Here's how the part is built. I have some questions about the finished solid (model axes, mm). Face numbers are marked on the shaded views. A direction names the side the tool comes from. Give positions to 0.01 mm unless a question says otherwise; leave off trailing zeros. Write each loop counter-clockwise with the first axis right and the second up, starting at its lowest first coordinate (ties: lowest second). Pieces come first, ordered by that corner, then holes. Notation, with made-up numbers: (16, 21) -> (32, 21) arc R26 ccw to (32, 49) -> close; hole circle Ø10 at (33.25, -8.5). An arc over 180 degrees is marked (long way). Return JSON: item names as keys, results as strings.
from build123d import *

# Parameters (mm, degrees)
SKETCH1_R               = 10
BOSS_EXTRUDE1_DEPTH     = 115
SKETCH2_R               = 5
BOSS_EXTRUDE2_DEPTH     = 25
SKETCH3_R               = 5
CUT_EXTRUDE1_DEPTH      = 110
SKETCH4_R               = 2.5
CUT_EXTRUDE2_DEPTH      = 11
CUT_EXTRUDE2_DEPTH_BACK = 11
SKETCH5_R               = 10
BOSS_EXTRUDE3_DEPTH     = 22
SKETCH6_W               = 21
SKETCH6_H               = 21
BOSS_EXTRUDE4_DEPTH     = 8
SKETCH7_W               = 21
SKETCH7_H               = 21
BOSS_EXTRUDE5_DEPTH     = 2
SKETCH8_R               = 5
SKETCH8_R_2             = 4
CUT_EXTRUDE3_DEPTH      = 2
SKETCH9_R               = 1.545135807
CUT_EXTRUDE4_DEPTH      = 2


with BuildPart() as part:
    # Sketch1 → Boss-Extrude1 (new body)
    with BuildSketch(Plane.XY):
        Circle(SKETCH1_R)
    extrude(amount=BOSS_EXTRUDE1_DEPTH)

    # Sketch2 → Boss-Extrude2 (add)
    with BuildSketch(Plane(origin=(0, 0, 0), x_dir=(-1, 0, 0), z_dir=(0, 0, -1))):
        Circle(SKETCH2_R)
    extrude(amount=BOSS_EXTRUDE2_DEPTH)

    # Sketch3 → Cut-Extrude1 (cut)
    with BuildSketch(Plane.XY.offset(115)):
        Circle(SKETCH3_R)
    extrude(amount=-CUT_EXTRUDE1_DEPTH, mode=Mode.SUBTRACT)

    # Sketch4 → Cut-Extrude2 (cut, two sides)
    with BuildSketch(Plane(origin=(0, 0, 0), x_dir=(0, 0, -1), z_dir=(1, 0, 0))) as cut_extrude2_sk:
        with Locations((20, 0)):
            Circle(SKETCH4_R)
    extrude(amount=CUT_EXTRUDE2_DEPTH, mode=Mode.SUBTRACT)
    extrude(cut_extrude2_sk.sketch, amount=-CUT_EXTRUDE2_DEPTH_BACK, mode=Mode.SUBTRACT)

    # Sketch5 → Boss-Extrude3 (add)
    with BuildSketch(Plane(origin=(0, 0, 0), x_dir=(-1, 0, 0), z_dir=(0, 0, -1))):
        Polygon((0, -12.701705922), (11, -6.350852961), (11, 6.350852961), (0, 12.701705922), (-11, 6.350852961), (-11, -6.350852961), align=None)
        Circle(SKETCH5_R, mode=Mode.SUBTRACT)
    extrude(amount=-BOSS_EXTRUDE3_DEPTH)



with BuildPart() as body_2:
    # Sketch6 → Boss-Extrude4 (new body)
    with BuildSketch(Plane.ZY.offset(11)):
        with Locations((32.5, 2.201705922)):
            Rectangle(SKETCH6_W, SKETCH6_H)
    extrude(amount=BOSS_EXTRUDE4_DEPTH)


with BuildPart() as part_1:
    add(part.part)

    add(body_2.part)  # Boss-Extrude5 merges body 2
    # Sketch7 → Boss-Extrude5 (add)
    with BuildSketch(Plane(origin=(-11, 0, 0), x_dir=(0, 0, -1), z_dir=(1, 0, 0))):
        with Locations((-32.5, 2.201705922)):
            Rectangle(SKETCH7_W, SKETCH7_H)
    extrude(amount=BOSS_EXTRUDE5_DEPTH)

    # Sketch8 → Cut-Extrude3 (cut)
    with BuildSketch(Plane.ZY.offset(19)):
        with Locations((36.5, 6.201705922)):
            Circle(SKETCH8_R)
        with Locations((36.5, 6.201705922)):
            Circle(SKETCH8_R_2, mode=Mode.SUBTRACT)
    extrude(amount=-CUT_EXTRUDE3_DEPTH, mode=Mode.SUBTRACT)

    # Sketch9 → Cut-Extrude4 (cut)
    with BuildSketch(Plane.ZY.offset(19)):
        with Locations((36.5, 6.201705922)):
            Circle(SKETCH9_R)
    extrude(amount=-CUT_EXTRUDE4_DEPTH, mode=Mode.SUBTRACT)


solid = part_1.part
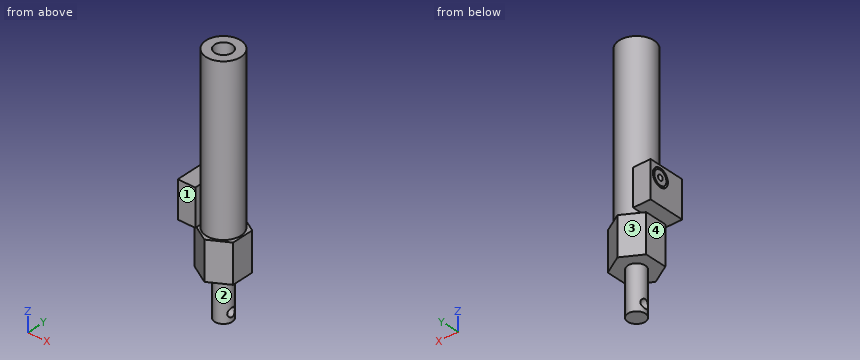
1. Suppose I cut it at A-A, the plane y = 0. List the corners of the cut face in (x, z) for me, and give its area (3 significant figures).
Taken from the geometry:
{"outline": "(-19, 22) -> (-11, 22) -> (-11, 0) -> (-5, 0) -> (-5, -17.5) -> (5, -17.5) -> (5, 0) -> (11, 0) -> (11, 22) -> (10, 22) -> (10, 115) -> (5, 115) -> (5, 5) -> (-5, 5) -> (-5, 115) -> (-10, 115) -> (-10, 43) -> (-19, 43) -> close; (-5, -25) -> (5, -25) -> (5, -22.5) -> (-5, -22.5) -> close", "area": "1,630 mm²"}
2. If I drill on line 1 (Y direction, x = -17.6, z = 36.5); line 2 (Y direction, x = -0.5, z = -20); line 3 (Y direction, x = -2.5, z = -20), over which ranges is the centre line in solid material (lowest first)? Write a range as [from, to].
Taken from the geometry:
{"line 1": "y = [-8.3, 1.2], [2.2, 4.66], [7.75, 10.2], [11.2, 12.7]", "line 2": "y = [-4.97, -2.5], [2.5, 4.97]", "line 3": "y = [-4.33, -2.5], [2.5, 4.33]"}
3. Suppose I cut it at B-B, the plane z = 36.5. List the corners of the cut face in (x, y) for me, and give its area (3 significant figures).
Taken from the geometry:
{"outline": "(-19, -8.3) -> (-9, -8.3) -> (-9, -4.36) arc R10 ccw (long way) to (-9, 4.36) -> (-9, 12.7) -> (-19, 12.7) -> (-19, 11.2) -> (-17, 11.2) -> (-17, 10.2) -> (-19, 10.2) -> (-19, 7.75) -> (-17, 7.75) -> (-17, 4.66) -> (-19, 4.66) -> (-19, 2.2) -> (-17, 2.2) -> (-17, 1.2) -> (-19, 1.2) -> close; hole circle Ø10 at (0, 0)", "area": "430 mm²"}
4. For pin 1 Ø2.5 at (y, z) = (6.2, 36.5) entering from -X; pin 2 Ø5 at (y, z) = (6, -7.5) entering from +X; pin 3 Ø3 at (y, z) = (-10, 14) entering from -X, each with a flat end and sliding along its axis, tell me the tip position at first contact or that it passes through.
Taken from the geometry:
{"pin 1": "stops at x = -17", "pin 2": "stops at x = 3.57", "pin 3": "stops at x = -7.28"}
5. Which directions (+Z, -Z, +X, -X, +Y, -Y) give clear straight access to the entire face, cutting with the end or side of a thin tool? Please do the marked faces 1, 2, 3 and 4.
Taken from the geometry:
{"face 1": "+Z, -Z, -X, -Y", "face 2": "-Z", "face 3": "-Z, -X, +Y", "face 4": "-Z, -X, +Y, -Y"}
6. Suppose I cut it at D-D, the plane z = -20. List the corners of the cut face in (x, y) for me, and give its area (3 significant figures).
Taken from the geometry:
{"outline": "(-4.33, -2.5) arc R5 ccw to (4.33, -2.5) -> close; (-4.33, 2.5) -> (4.33, 2.5) arc R5 ccw to start", "area": "30.7 mm²"}
7. Suppose I cut it at C-C, the plane x = -6.5. List the corners of the cut face in (y, z) for me, and give its area (3 significant figures).
Taken from the geometry:
{"outline": "(-8.95, 0) -> (8.95, 0) -> (8.95, 22) -> (7.6, 22) -> (7.6, 115) -> (-7.6, 115) -> (-7.6, 22) -> (-8.95, 22) -> close", "area": "1,810 mm²"}
